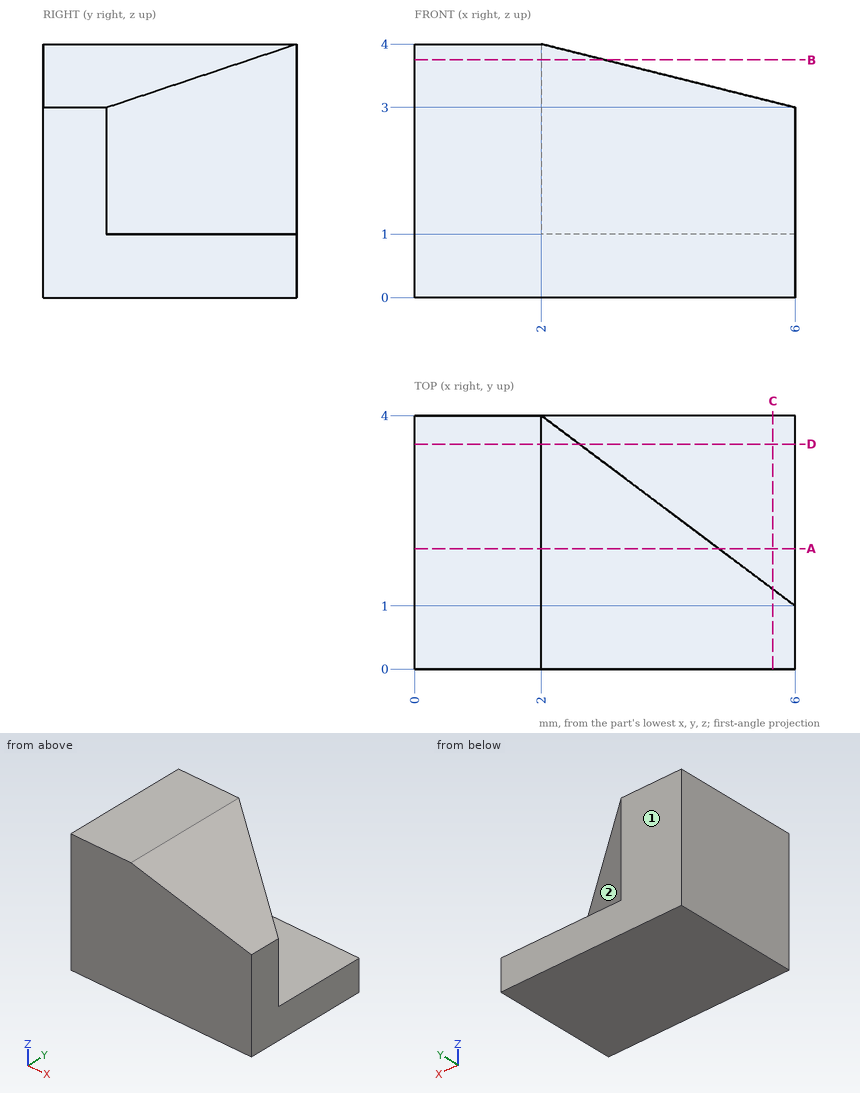
Answer from the drawing. Dimensions are ordinates in mm from the lowest x, y and z of the part. A direction names the side the tool comes from. Coordinates: 2 decimals unless noted, no trailing zeros. Loops run counter-clockwise (first coordinate to the right, second up) from the corner with the lowest first, then second, coordinate; pieces in that order, holes last.
1) Section A-A (y = 1.9) is taken. Give the vertices of the cut face in (x, z).
Results:
outline: (0, 0) - (6, 0) - (6, 1) - (4.8, 1) - (4.8, 3.3) - (2, 4) - (0, 4) - close
2) For the marked faces 1 and 2, determine the directions among +Z, -Z, +X, -X, +Y, -Y from which every point of the face is accessible in a straight line to the end or side of a thin tool.
Results:
face 1: +Z, -Z, +X, -X, +Y
face 2: +Z, +X, +Y
3) Section D-D (y = 3.55) is taken. Give the vertices of the cut face in (x, z).
Results:
outline: (0, 0) - (6, 0) - (6, 1) - (2.6, 1) - (2.6, 3.85) - (2, 4) - (0, 4) - close
4) Section B-B (z = 3.75) is taken. Give the vertices of the cut face in (x, y), plus the area to 3 significant figures.
Results:
outline: (0, 0) - (3, 0) - (3, 3.25) - (2, 4) - (0, 4) - close
area: 11.6 mm2
5) Flat-ended cylindrical pins translate along their axes: pin 1 (2 mm diameter, centred on x = 3.5, y = 3.5, fed in from +Z) (3 decimals); pin 2 (0.9 mm diameter, centred on x = 4.5, y = 2.5, fed in from +Z). Find the tip coordinate at first contact, or state that the pin passes through.
Results:
pin 1: stops at z = 3.875
pin 2: stops at z = 3.49
6) Consider probe 1 along Z at (x, y) = (5.45, 2.8); probe 2 along Z at (x, y) = (3.85, 0.4); probe 3 along Y at (x, z) = (2.9, 1.6) (3 decimals). Determine where each line is inside the solid, lowest interval first.
Results:
probe 1: z = 0 to 1
probe 2: z = 0 to 3.54
probe 3: y = 0 to 3.325
7) Section C-C (x = 5.65) is taken. Give the vertices of the cut face in (y, z), plus the area to 3 significant figures.
Results:
outline: (0, 0) - (4, 0) - (4, 1) - (1.26, 1) - (1.26, 3.09) - (0, 3.09) - close
area: 6.64 mm2
